Autodesk Inventor part; units mm, degrees
ref_plane "YZ Plane" through (0, 0, 0) normal (1, 0, 0) x (0, 1, 0)
ref_plane "XZ Plane" through (0, 0, 0) normal (0, 1, 0) x (-1, 0, 0)
ref_plane "XY Plane" through (0, 0, 0) normal (0, 0, 1) x (1, 0, 0)
sketch "Sketch1" plane through (0, 0, 0) normal (0, 0, 1) x (1, 0, 0)
  line L0 (0, 0) -> (25.4, 0)
  line L1 (25.4, 0) -> (25.4, -101.6)
  line L2 (25.4, -101.6) -> (0, -101.6)
  line L3 (0, -101.6) -> (0, 0)
  line L4 (22.225, -3.175) -> (3.175, -3.175)
  line L5 (3.175, -3.175) -> (3.175, -98.425)
  line L6 (3.175, -98.425) -> (22.225, -98.425)
  line L7 (22.225, -98.425) -> (22.225, -3.175)
  dimension "d0" = 25.4
  dimension "d1" = 101.6
  dimension "d2" = 3.175
extrude "Extrusion1" add sketch "Sketch1" along normal blind 1016
sketch "Sketch2" plane through (25.4, -101.6, 0) normal (1, 0, 0) x (0, 0, -1)
  point P0 (0, 101.6)
  point P1 (-114.3, 25.4)
sketch "Sketch3" plane through (25.4, -101.6, 0) normal (1, 0, 0) x (0, 0, -1)
  point P0 (0, 101.6)
  point P1 (-901.7, 25.4)
hole "Hole1" at (25.4, -76.2, 901.7) direction (-1, 0, 0) diameter 9.525 end through all
hole "Hole2" at (25.4, -76.2, 114.3) direction (-1, 0, 0) diameter 9.525 end through all
properties part number "4x1 boxbeam"
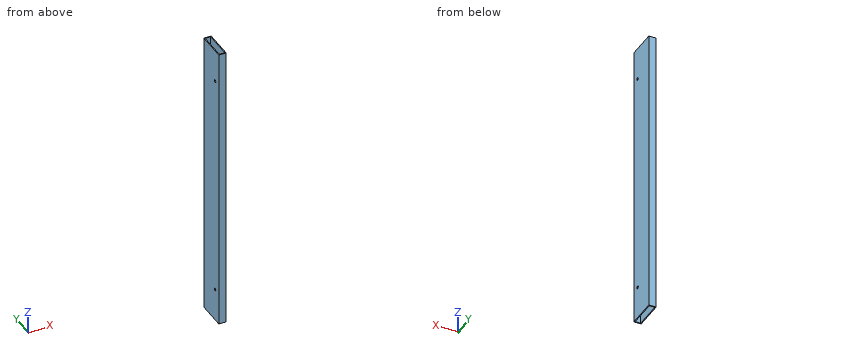
The model under review builds one solid part; all positions refer to its coordinate system, in mm. Coordinates: 2 decimals unless noted, no trailing zeros. Write each loop counter-clockwise with the first axis right and the second up, starting at its lowest first coordinate (ties: lowest second). Pieces come first, ordered by that corner, then holes. Notation, with made-up numbers: (63.25, 75.25) -> (85.25, 75.25) arc R29 ccw to (85.25, 114.25) -> close; hole circle Ø11 at (12.25, 28.25). An arc over 180 degrees is marked (long way). One line per item, written item: value. Start each with the question number.
Q1. Add section A-A, the plane y = -22.5. Give the boundary of the cut face in (x, z) (3 decimals).
Q2. To check wall thickness, follow probe 1 along Z at (x, y) = (22.95, -76.2); probe 2 along Y at (x, z) = (1.05, 901.7); probe 3 along X at (y, z) = (-6.5, 65.5) (3 decimals). State the ranges of each line that lie inside material, in increasing order.
Q3. Add section B-B, the plane z = 139.5. Give the boundary of the cut face in (x, y) (3 decimals).
Q4. Clearance check with a flat-ended pin moving along its axis: P1, Ø7.5, axis at y = -76.2, z = 114.3, coming from the -X side. State where the tip first meets the part, or that it passes through.
Response:
1. outline: (0, 0) -> (3.175, 0) -> (3.175, 1016) -> (0, 1016) -> close; (22.225, 0) -> (25.4, 0) -> (25.4, 1016) -> (22.225, 1016) -> close
2. probe 1: 0 to 109.54, 119.06 to 896.94, 906.46 to 1016
2. probe 2: -101.6 to -80.96, -71.44 to 0
2. probe 3: 0 to 3.175, 22.225 to 25.4
3. outline: (0, -101.6) -> (25.4, -101.6) -> (25.4, 0) -> (0, 0) -> close; hole (3.175, -98.425) -> (22.225, -98.425) -> (22.225, -3.175) -> (3.175, -3.175) -> close
4. P1: through
